Work out the finished part from the listing and answer in its coordinate system (mm). Give positions to 0.01 mm unless a question says otherwise; leave off trailing zeros. Loops run counter-clockwise (first coordinate to the right, second up) from the corner with the lowest first, then second, coordinate; pieces in that order, holes last. Notation, with made-up numbers: M 16.25,13.5 L 66.25,13.5 A6 ccw 66.25,19.5 Z; hole C 76,84.25 d5. An arc over 180 degrees is marked long. Write item = value, one per line. Start each with the question number.
1. Flat-ended cylindrical pins translate along their axes: pin 1 Ø3 at (y, z) = (1, -20.5) entering from +X; pin 2 Ø1.5 at (x, y) = (-6, 1) entering from -Z; pin 3 Ø2 at (y, z) = (3.5, 33.5) entering from +X; pin 4 Ø12 at (x, z) = (-10, 12.5) entering from +Y. Find the tip coordinate at first contact, or state that the pin passes through.
2. Section A-A on x = 0 is taken. Determine the outline of the cut face in (y, z), plus the area to 3 significant figures.
3. Section B-B on z = 0 is taken. Give the number of separate pieces and of enclosed holes in the cut face, plus the area to 3 significant figures.
4. The mould has two halves that part along X. Classify faces 1 (the face through (22.34, 2.46, 13.3)), 2 (the face through (1.106, 2.465, 10.181)), 3 (the face through (1, 5, 1)): released by +X, released by -X, zero draft, split by the parting line, or undercut.
5. Consider L1, parallel to Z at x = -15, y = 2.3 (3 decimals); L2, parallel to Z at x = 21, y = 2.5; L3, parallel to Z at x = -27, y = 2. Determine where each line is inside the solid, lowest interval first. Write a range as [from, to].
6. Section C-C on x = 34 is taken. Determine the outline of the cut face in (y, z).
```python
from build123d import *

# Parameters (mm, degrees)
MODEL_R                         = 42.5
AUFSATZ_LINEAR_AUSTRAGEN1_DEPTH = 5


with BuildPart() as part:
    # Model → Aufsatz-Linear austragen1 (new body)
    with BuildSketch(Plane.XZ):
        with Locations(Location((0, 0, 0), (0, 0, 270))):  # turned: the seam where the file's is
            Circle(MODEL_R)
        with BuildLine():
            ThreePointArc((4.5, -3.968626967), (6, 0), (4.5, 3.968626967))
            ThreePointArc((4.5, 3.968626967), (1.677124344, 4.145751311), (1.5, 1.322875656))
            ThreePointArc((1.5, 1.322875656), (2, 0), (1.5, -1.322875656))
            ThreePointArc((1.5, -1.322875656), (1.677124344, -4.145751311), (4.5, -3.968626967))
        make_face(mode=Mode.SUBTRACT)
        with BuildLine():
            ThreePointArc((-1.5, 1.322875656), (-1.677124344, 4.145751311), (-4.5, 3.968626967))
            ThreePointArc((-4.5, 3.968626967), (-6, 0), (-4.5, -3.968626967))
            ThreePointArc((-4.5, -3.968626967), (-1.677124344, -4.145751311), (-1.5, -1.322875656))
            ThreePointArc((-1.5, -1.322875656), (-2, 0), (-1.5, 1.322875656))
        make_face(mode=Mode.SUBTRACT)
        with BuildLine():
            ThreePointArc((-5.409084657, -5.894217775), (-8.234910265, -6.015501054), (-8.113626985, -8.841326662))
            ThreePointArc((-8.113626985, -8.841326662), (0, -12), (8.113626985, -8.841326662))
            ThreePointArc((8.113626985, -8.841326662), (8.234910265, -6.015501054), (5.409084657, -5.894217775))
            ThreePointArc((5.409084657, -5.894217775), (0, -8), (-5.409084657, -5.894217775))
        make_face(mode=Mode.SUBTRACT)
        with BuildLine():
            ThreePointArc((7.809084657, -1.737295837), (9.327031862, -4.12389096), (11.713626985, -2.605943755))
            ThreePointArc((11.713626985, -2.605943755), (10.392304845, 6), (3.6, 11.447270417))
            ThreePointArc((3.6, 11.447270417), (1.092121597, 10.139392014), (2.4, 7.631513611))
            ThreePointArc((2.4, 7.631513611), (6.92820323, 4), (7.809084657, -1.737295837))
        make_face(mode=Mode.SUBTRACT)
        with BuildLine():
            ThreePointArc((-10.59682539, -9.149168905), (-13.417681718, -8.942360836), (-13.624489787, -11.763217163))
            ThreePointArc((-13.624489787, -11.763217163), (0, -18), (13.624489787, -11.763217163))
            ThreePointArc((13.624489787, -11.763217163), (13.417681718, -8.942360836), (10.59682539, -9.149168905))
            ThreePointArc((10.59682539, -9.149168905), (0, -14), (-10.59682539, -9.149168905))
        make_face(mode=Mode.SUBTRACT)
        with BuildLine():
            ThreePointArc((13.22182539, -4.602535535), (14.453152512, -7.14887281), (16.999489787, -5.917545688))
            ThreePointArc((16.999489787, -5.917545688), (15.588457268, 9), (3.375, 17.680762851))
            ThreePointArc((3.375, 17.680762851), (1.035470794, 16.091233646), (2.625, 13.75170444))
            ThreePointArc((2.625, 13.75170444), (12.124355653, 7), (13.22182539, -4.602535535))
        make_face(mode=Mode.SUBTRACT)
        with BuildLine():
            ThreePointArc((-3.214285714, 29.827309087), (-25.980762114, 15), (-27.438350253, -12.13000146))
            ThreePointArc((-27.438350253, -12.13000146), (-24.800460139, -13.150558046), (-23.779903552, -10.512667932))
            ThreePointArc((-23.779903552, -10.512667932), (-22.516660498, 13), (-2.785714286, 25.850334542))
            ThreePointArc((-2.785714286, 25.850334542), (-1.011512728, 28.053107528), (-3.214285714, 29.827309087))
        make_face(mode=Mode.SUBTRACT)
        with BuildLine():
            ThreePointArc((-22.226821187, -9.053641252), (-19.620115984, -10.151406246), (-18.522350989, -7.544701043))
            ThreePointArc((-18.522350989, -7.544701043), (-17.320508076, 10), (-2.727272727, 19.813177016))
            ThreePointArc((-2.727272727, 19.813177016), (-1.018682298, 22.06722199), (-3.272727273, 23.775812419))
            ThreePointArc((-3.272727273, 23.775812419), (-20.784609691, 12), (-22.226821187, -9.053641252))
        make_face(mode=Mode.SUBTRACT)
        with BuildLine():
            ThreePointArc((-2.4, 7.631513611), (-1.092121597, 10.139392014), (-3.6, 11.447270417))
            ThreePointArc((-3.6, 11.447270417), (-10.392304845, 6), (-11.713626985, -2.605943755))
            ThreePointArc((-11.713626985, -2.605943755), (-9.327031862, -4.12389096), (-7.809084657, -1.737295837))
            ThreePointArc((-7.809084657, -1.737295837), (-6.92820323, 4), (-2.4, 7.631513611))
        make_face(mode=Mode.SUBTRACT)
        with BuildLine():
            ThreePointArc((-2.625, 13.75170444), (-1.035470794, 16.091233646), (-3.375, 17.680762851))
            ThreePointArc((-3.375, 17.680762851), (-15.588457268, 9), (-16.999489787, -5.917545688))
            ThreePointArc((-16.999489787, -5.917545688), (-14.453152512, -7.14887281), (-13.22182539, -4.602535535))
            ThreePointArc((-13.22182539, -4.602535535), (-12.124355653, 7), (-2.625, 13.75170444))
        make_face(mode=Mode.SUBTRACT)
        with BuildLine():
            ThreePointArc((27.438350253, -12.13000146), (25.980762114, 15), (3.214285714, 29.827309087))
            ThreePointArc((3.214285714, 29.827309087), (1.011512728, 28.053107528), (2.785714286, 25.850334542))
            ThreePointArc((2.785714286, 25.850334542), (22.516660498, 13), (23.779903552, -10.512667932))
            ThreePointArc((23.779903552, -10.512667932), (24.800460139, -13.150558046), (27.438350253, -12.13000146))
        make_face(mode=Mode.SUBTRACT)
        with BuildLine():
            ThreePointArc((-24.224064538, -17.697307627), (0, -30), (24.224064538, -17.697307627))
            ThreePointArc((24.224064538, -17.697307627), (23.788947411, -14.902549483), (20.994189267, -15.33766661))
            ThreePointArc((20.994189267, -15.33766661), (0, -26), (-20.994189267, -15.33766661))
            ThreePointArc((-20.994189267, -15.33766661), (-23.788947411, -14.902549483), (-24.224064538, -17.697307627))
        make_face(mode=Mode.SUBTRACT)
        with BuildLine():
            ThreePointArc((3.272727273, 23.775812419), (1.018682298, 22.06722199), (2.727272727, 19.813177016))
            ThreePointArc((2.727272727, 19.813177016), (17.320508076, 10), (18.522350989, -7.544701043))
            ThreePointArc((18.522350989, -7.544701043), (19.620115984, -10.151406246), (22.226821187, -9.053641252))
            ThreePointArc((22.226821187, -9.053641252), (20.784609691, 12), (3.272727273, 23.775812419))
        make_face(mode=Mode.SUBTRACT)
        with BuildLine():
            ThreePointArc((18.954093914, -14.722171167), (18.601433685, -11.915815744), (15.795078262, -12.268475973))
            ThreePointArc((15.795078262, -12.268475973), (0, -20), (-15.795078262, -12.268475973))
            ThreePointArc((-15.795078262, -12.268475973), (-18.601433685, -11.915815744), (-18.954093914, -14.722171167))
            ThreePointArc((-18.954093914, -14.722171167), (0, -24), (18.954093914, -14.722171167))
        make_face(mode=Mode.SUBTRACT)
    extrude(amount=-AUFSATZ_LINEAR_AUSTRAGEN1_DEPTH)


solid = part.part
```
Verdict:
q1.pin_1 = 38.02
q1.pin_2 = -42.17
q1.pin_3 = 27.39
q1.pin_4 = 5
q2.outline = M 0,-42.5 L 5,-42.5 L 5,-30 L 0,-30 Z; M 0,-26 L 5,-26 L 5,-24 L 0,-24 Z; M 0,-20 L 5,-20 L 5,-18 L 0,-18 Z; M 0,-14 L 5,-14 L 5,-12 L 0,-12 Z; M 0,-8 L 5,-8 L 5,42.5 L 0,42.5 Z
q2.area = 345 mm2
q3.separate_pieces = 11
q3.enclosed_holes = 0
q3.area = 225 mm2
q4.face_1 = undercut
q4.face_2 = undercut
q4.face_3 = zero draft
q5.L1 = [-39.765, -25.981], [-21.237, -18.735], [-13.229, -7.257], [9.95, 13.229], [18.735, 21.237], [25.981, 39.765]
q5.L2 = [-36.95, -21.42], [-15.33, -10.2], [11.62, 15.33], [21.42, 36.95]
q5.L3 = [-32.82, -12.76], [13.08, 32.82]
q6.outline = M 0,-25.5 L 5,-25.5 L 5,25.5 L 0,25.5 Z
